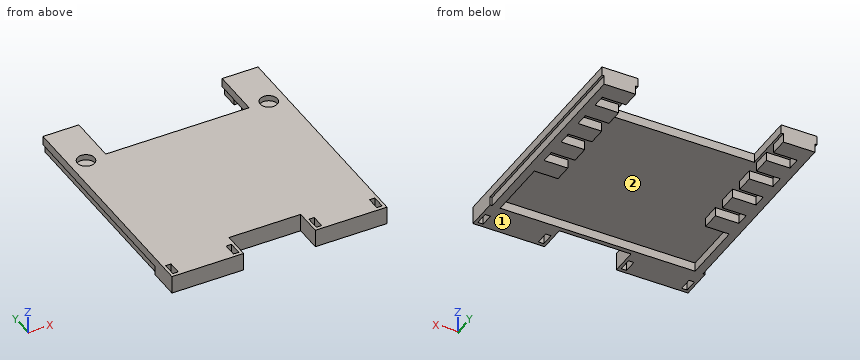
```python
from build123d import *

# Parameters (mm, degrees)
BASE_DEPTH              = 3.175
SECOND_LAYER_DEPTH      = 3.175
SKETCH6_R               = 3.048
MAGNET_HOLDER_DEPTH     = 2
SKETCH7_W               = 1.905
SKETCH7_H               = 4.74726
SMALL_MAGNETS_CUT_DEPTH = 6.35


with BuildPart() as part:
    # Sketch1 → base (new body)
    with BuildSketch(Plane.XY):
        Polygon((88.9, -120.65), (88.9, -36.83), (76.2, -36.83), (76.2, -54.2925), (25.4, -54.2925), (25.4, -36.83), (12.7, -36.83), (12.7, -120.65), (38.1, -120.65), (38.1, -111.125), (63.5, -111.125), (63.5, -120.65), align=None)
    extrude(amount=-BASE_DEPTH)

    # Sketch2 → second layer (add)
    with BuildSketch(Plane(origin=(0, 0, -3.175), x_dir=(-1, 0, 0), z_dir=(0, 0, -1))):
        Polygon((-88.9, -120.65), (-88.9, -109.5375), (-88.138, -109.5375), (-88.138, -36.83), (-76.962, -36.83), (-76.962, -43.18), (-85.344, -43.18), (-85.344, -47.863125), (-76.962, -47.863125), (-76.962, -54.213125), (-85.344, -54.213125), (-85.344, -58.89625), (-76.962, -58.89625), (-76.962, -65.24625), (-85.344, -65.24625), (-85.344, -69.929375), (-76.962, -69.929375), (-76.962, -76.279375), (-85.344, -76.279375), (-85.344, -80.9625), (-76.962, -80.9625), (-76.962, -87.3125), (-85.344, -87.3125), (-85.344, -109.5375), (-16.256, -109.5375), (-16.256, -87.3125), (-24.638, -87.3125), (-24.638, -80.9625), (-16.256, -80.9625), (-16.256, -76.279375), (-24.638, -76.279375), (-24.638, -69.929375), (-16.256, -69.929375), (-16.256, -65.24625), (-24.638, -65.24625), (-24.638, -58.89625), (-16.256, -58.89625), (-16.256, -54.213125), (-24.638, -54.213125), (-24.638, -47.863125), (-16.256, -47.863125), (-16.256, -43.18), (-24.638, -43.18), (-24.638, -36.83), (-13.462, -36.83), (-13.462, -109.5375), (-12.7, -109.5375), (-12.7, -120.65), (-38.1, -120.65), (-38.1, -111.125), (-63.5, -111.125), (-63.5, -120.65), align=None)
    extrude(amount=SECOND_LAYER_DEPTH)

    # Sketch6 → magnet holder (cut)
    with BuildSketch(Plane.XY):
        with Locations((18.415, -54.2925)):
            Circle(SKETCH6_R)
        with Locations(Location((83.185, -54.2925, 0), (0, 0, 180))):  # turned: the seam where the file's is
            Circle(SKETCH6_R)
    extrude(amount=-MAGNET_HOLDER_DEPTH, mode=Mode.SUBTRACT)

    # Sketch7 → small magnets cut (cut)
    with BuildSketch(Plane.XY):
        with Locations((14.6685, -117.00637)):
            Rectangle(SKETCH7_W, SKETCH7_H)
        with Locations((36.1315, -117.00637)):
            Rectangle(SKETCH7_W, SKETCH7_H)
        with Locations((65.4685, -117.00637)):
            Rectangle(SKETCH7_W, SKETCH7_H)
        with Locations((86.9315, -117.00637)):
            Rectangle(SKETCH7_W, SKETCH7_H)
    extrude(amount=-SMALL_MAGNETS_CUT_DEPTH, mode=Mode.SUBTRACT)


solid = part.part
```
Geometry: final body of the model. Coordinates: model frame, mm. Face numbers are marked on the shaded views. Coordinates: 2 decimals unless noted, no trailing zeros. Write each loop counter-clockwise with the first axis right and the second up, starting at its lowest first coordinate (ties: lowest second). Pieces come first, ordered by that corner, then holes. Notation, with made-up numbers: M 13.5,19.25 L 65.5,19.25 A22 ccw 65.5,49.25 Z; hole C 63,-27.75 d3. An arc over 180 degrees is marked long. Use CSV: the item, a comma, the result in double quotes. Start each with the question number.
1. First-contact query: P1, Ø1, axis at x = 46, y = -64, coming from the -Z side (3 decimals); P2, Ø3, axis at x = 52, z = -3.5, coming from the -Y side (3 decimals); P3, Ø1, axis at y = -78.5, z = -4.5, coming from the +X side. Flat tips, straight axial feed; report the tip coordinate or a pass-through.
2. Mould query, pull axis X, two halves, no side actions, for the marked faces 1 and 2. Classes: pulls with the +X half, pulls with the -X half, needs draft (parallel to the pull), parting line crosses it, or undercut.
3. Cut plane D-D on y = -82.5. Return the cut outline in (x, z) (3 decimals).
4. Cut plane A-A on y = -91. Return the cut outline in (x, z) (3 decimals).
5. Ray query, probe 1 along X at (y, z) = (-115.5, -4.25); probe 2 along Y at (x, z) = (23.5, -3.25); probe 3 along X at (y, z) = (-92.5, -5.25). Return the intervals inside material, ascending.
6. Cut plane C-C on z = -4.5. Count the separate pieces of the cut face and the enclosed holes in it, plus the area to 3 significant figures.
Entries:
1,P1,"z = -3.175"
1,P2,"y = -111.125"
1,P3,"x = 88.14"
2,face 1,"needs draft"
2,face 2,"undercut"
3,outline,"M 12.7,-3.175 L 13.462,-3.175 L 13.462,-6.35 L 24.638,-6.35 L 24.638,-3.175 L 76.962,-3.175 L 76.962,-6.35 L 88.138,-6.35 L 88.138,-3.175 L 88.9,-3.175 L 88.9,0 L 12.7,0 Z"
4,outline,"M 12.7,-3.175 L 13.462,-3.175 L 13.462,-6.35 L 16.256,-6.35 L 16.256,-3.175 L 85.344,-3.175 L 85.344,-6.35 L 88.138,-6.35 L 88.138,-3.175 L 88.9,-3.175 L 88.9,0 L 12.7,0 Z"
5,probe 1,"12.7 to 13.72, 15.62 to 35.18, 37.08 to 38.1, 63.5 to 64.52, 66.42 to 85.98, 87.88 to 88.9"
5,probe 2,"-120.65 to -109.54, -87.31 to -80.96, -76.28 to -69.93, -65.25 to -58.9, -54.21 to -47.86, -43.18 to -36.83"
5,probe 3,"13.46 to 16.26, 85.34 to 88.14"
6,separate pieces,"1"
6,enclosed holes,"4"
6,area,"1,510 mm²"
